```python
from build123d import *

# Parameters (mm, degrees)
SKETCH2_W                    = 33.9
SKETCH2_H                    = 1
BASE_FLANGE1_DEPTH           = 2000
EDGE_FLANGE2_STRIP_W         = 5.4732
EDGE_FLANGE2_STRIP_H         = 1
EDGE_FLANGE2_STRIP_CUT_DEPTH = 2000
EDGE_FLANGE2_DEPTH           = 2000
SKETCH10_R                   = 3
CUT_EXTRUDE1_DEPTH           = 10
SKETCH10_3_R                 = 3
CUT_EXTRUDE2_DEPTH           = 10


# Sheet-metal steps are written as plain solids
with BuildPart() as part:
    # Sketch2 → Base-Flange1 (new body)
    with BuildSketch(Plane(origin=(0, 0, 0), x_dir=(0, 0, -1), z_dir=(1, 0, 0))):
        with Locations((16.95, -0.5)):
            Rectangle(SKETCH2_W, SKETCH2_H)
    extrude(amount=BASE_FLANGE1_DEPTH)

    # Edge-Flange2 strip (across the edge) → Edge-Flange2 strip cut (cut)
    with BuildSketch(Plane(origin=(2000, 0, -33.9), x_dir=(0, 0, 1), z_dir=(-1, 0, 0))):
        with Locations((-1, -0.5)):
            Rectangle(EDGE_FLANGE2_STRIP_W, EDGE_FLANGE2_STRIP_H)
    extrude(amount=EDGE_FLANGE2_STRIP_CUT_DEPTH, mode=Mode.SUBTRACT)

    # Edge-Flange2 section (across the edge) → Edge-Flange2 (add)
    with BuildSketch(Plane(origin=(2000, 0, -33.9), x_dir=(0, 0, 1), z_dir=(-1, 0, 0))):
        with BuildLine():
            Line((0, 0.7366), (0, 149))
            Line((0, 149), (1, 149))
            Line((1, 149), (1, 0.7366))
            ThreePointArc((1, 0.7366), (1.215745145, 0.215745145), (1.7366, 0))
            Line((1.7366, 0), (1.7366, -1))
            ThreePointArc((1.7366, -1), (0.508638364, -0.491361636), (0, 0.7366))
        make_face()
    extrude(amount=EDGE_FLANGE2_DEPTH)

    # Sketch10 → Cut-Extrude1 (cut)
    with BuildSketch(Plane(origin=(0, 0, 0), x_dir=(1, 0, 0), z_dir=(0, 1, 0))):
        with Locations(Location((860, 16.95, 0), (0, 0, 270))):
            Circle(SKETCH10_R)
    extrude(amount=-CUT_EXTRUDE1_DEPTH, mode=Mode.SUBTRACT)

    # Sketch10<3> → Cut-Extrude2 (cut)
    with BuildSketch(Plane(origin=(0, 0, 0), x_dir=(1, 0, 0), z_dir=(0, 1, 0))):
        with Locations(Location((460, 16.95, 0), (0, 0, 270))):
            Circle(SKETCH10_3_R)
        with Locations(Location((860, 16.95, 0), (0, 0, 270))):
            Circle(SKETCH10_3_R)
        with Locations(Location((1260, 16.95, 0), (0, 0, 270))):
            Circle(SKETCH10_3_R)
        with Locations(Location((1660, 16.95, 0), (0, 0, 270))):
            Circle(SKETCH10_3_R)
    extrude(amount=-CUT_EXTRUDE2_DEPTH, mode=Mode.SUBTRACT)


solid = part.part
```
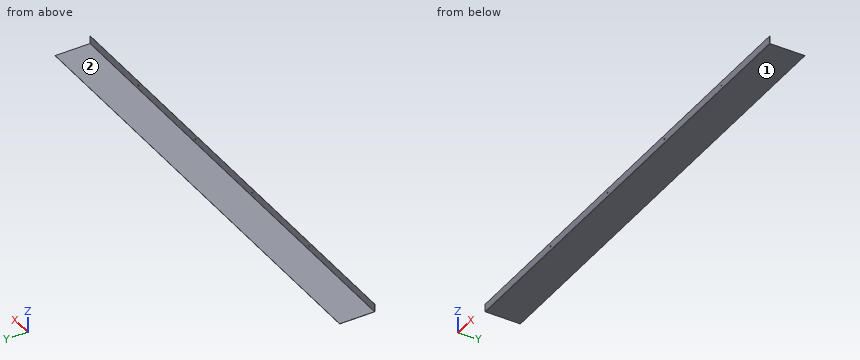
Verification items for the finished model (mm, model axes). Face numbers are marked on the shaded views. A direction names the side the tool comes from. Coordinates: 2 decimals unless noted, no trailing zeros. Loops run counter-clockwise (first coordinate to the right, second up) from the corner with the lowest first, then second, coordinate; pieces in that order, holes last. Notation, with made-up numbers: (-27.5, 5) - (-7.5, 5) arc R13 ccw to (-7.5, 22) - close; hole circle Ø10 at (33.5, 84). An arc over 180 degrees is marked (long way). Answer as a JSON object with one key per item and string values.
(1) Cross-section at C-C, the plane z = -5.5. Record the boundary of the cut face in (x, y).
Response:
{"outline": "(0, -1) - (2000, -1) - (2000, 0) - (0, 0) - close"}
(2) Access from +Z, -Z, +X, -X, +Y, -Y to the whole of each face (thin tool, end or side, straight path). Record for the marked faces 1 and 2.
Response:
{"face 1": "-Z, +X, -X, +Y, -Y", "face 2": "+Z, +X, -X, +Y"}
(3) Cross-section at A-A, the plane x = 791. Record the boundary of the cut face in (y, z).
Response:
{"outline": "(-1, -32.16) arc R1.74 ccw to (0.74, -33.9) - (149, -33.9) - (149, -32.9) - (0.74, -32.9) arc R0.74 cw to (0, -32.16) - (0, 0) - (-1, 0) - close"}
(4) Cross-section at B-B, the plane y = 39.5. Record the boundary of the cut face in (x, z), then the cut area to 3 significant figures.
Response:
{"outline": "(0, -33.9) - (2000, -33.9) - (2000, -32.9) - (0, -32.9) - close", "area": "2,000 mm²"}
(5) Go/stop test with flat-tipped pins: pin 1 Ø9.5 at (x, z) = (1015.5, -22) entering from +Y; pin 2 Ø6 at (x, y) = (397, 35) entering from +Z; pin 3 Ø8 at (x, z) = (860, -16.95) entering from -Y; pin 4 Ø5 at (y, z) = (57, -28) entering from -X. Record where each tip stops, or that it passes through.
Response:
{"pin 1": "stops at y = 0", "pin 2": "stops at z = -32.9", "pin 3": "stops at y = -1", "pin 4": "passes through"}
(6) Scan lines: line 1 along X through (y, z) = (-0.4, -16.95); line 2 along Z through (x, y) = (860, -0.25); line 3 along Y through (x, z) = (1639, -22). Record each from-to range of solid material in increasing order.
Response:
{"line 1": "x = 0 to 457, 463 to 857, 863 to 1257, 1263 to 1657, 1663 to 2000", "line 2": "z = -33.59 to -19.95, -13.95 to 0", "line 3": "y = -1 to 0"}
